```python
from build123d import *

# Parameters (mm, degrees)
SKETCH2_W           = 150
SKETCH2_H           = 260
BOSS_EXTRUDE1_DEPTH = 10
SKETCH3_R           = 3.125
CUT_EXTRUDE1_DEPTH  = 151.416089565
SKETCH4_R           = 5.5
CUT_EXTRUDE2_DEPTH  = 5
SKETCH5_R           = 3.5
CUT_EXTRUDE3_DEPTH  = 151.416089565


with BuildPart() as part:
    # Sketch2 → Boss-Extrude1 (new body)
    with BuildSketch(Plane(origin=(0, 0, 0), x_dir=(1, 0, 0), z_dir=(0, 1, 0))):
        Rectangle(SKETCH2_W, SKETCH2_H)
    extrude(amount=BOSS_EXTRUDE1_DEPTH)

    # Sketch3 → Cut-Extrude1 (cut, through all)
    with BuildSketch(Plane(origin=(0, 10, 0), x_dir=(1, 0, 0), z_dir=(0, 1, 0))):
        with Locations(Location((-54.447222151, -54.447222151, 0), (0, 0, 270))):
            Circle(SKETCH3_R)
        with Locations(Location((-43.840620434, -43.840620434, 0), (0, 0, 270))):
            Circle(SKETCH3_R)
        with Locations(Location((54.447222151, 54.447222151, 0), (0, 0, 270))):
            Circle(SKETCH3_R)
        with Locations(Location((43.840620434, 43.840620434, 0), (0, 0, 270))):
            Circle(SKETCH3_R)
        with Locations(Location((-54.447222151, 54.447222151, 0), (0, 0, 270))):
            Circle(SKETCH3_R)
        with Locations(Location((-43.840620434, 43.840620434, 0), (0, 0, 270))):
            Circle(SKETCH3_R)
        with Locations(Location((54.447222151, -54.447222151, 0), (0, 0, 270))):
            Circle(SKETCH3_R)
        with Locations(Location((43.840620434, -43.840620434, 0), (0, 0, 270))):
            Circle(SKETCH3_R)
    extrude(amount=-CUT_EXTRUDE1_DEPTH, mode=Mode.SUBTRACT)

    # Sketch4 → Cut-Extrude2 (cut, symmetric)
    with BuildSketch(Plane(origin=(0, 10, 0), x_dir=(1, 0, 0), z_dir=(0, 1, 0))):
        with Locations(Location((-43.840620434, -43.840620434, 0), (0, 0, 270))):
            Circle(SKETCH4_R)
        with Locations(Location((-54.447222151, -54.447222151, 0), (0, 0, 270))):
            Circle(SKETCH4_R)
        with Locations(Location((43.840620434, -43.840620434, 0), (0, 0, 270))):
            Circle(SKETCH4_R)
        with Locations(Location((54.447222151, -54.447222151, 0), (0, 0, 270))):
            Circle(SKETCH4_R)
        with Locations(Location((43.840620434, 43.840620434, 0), (0, 0, 270))):
            Circle(SKETCH4_R)
        with Locations(Location((54.447222151, 54.447222151, 0), (0, 0, 270))):
            Circle(SKETCH4_R)
        with Locations(Location((-43.840620434, 43.840620434, 0), (0, 0, 270))):
            Circle(SKETCH4_R)
        with Locations(Location((-54.447222151, 54.447222151, 0), (0, 0, 270))):
            Circle(SKETCH4_R)
    extrude(amount=CUT_EXTRUDE2_DEPTH, both=True, mode=Mode.SUBTRACT)

    # Sketch5 → Cut-Extrude3 (cut, through all)
    with BuildSketch(Plane(origin=(0, 10, 0), x_dir=(1, 0, 0), z_dir=(0, 1, 0))):
        with Locations(Location((-65, 115, 0), (0, 0, 270))):
            Circle(SKETCH5_R)
        with Locations(Location((-39.6, 115, 0), (0, 0, 270))):
            Circle(SKETCH5_R)
        with Locations(Location((-14.2, 115, 0), (0, 0, 270))):
            Circle(SKETCH5_R)
        with Locations(Location((11.2, 115, 0), (0, 0, 270))):
            Circle(SKETCH5_R)
        with Locations(Location((36.6, 115, 0), (0, 0, 270))):
            Circle(SKETCH5_R)
        with Locations(Location((62, 115, 0), (0, 0, 270))):
            Circle(SKETCH5_R)
        with Locations(Location((-65, -113.6, 0), (0, 0, 270))):
            Circle(SKETCH5_R)
        with Locations(Location((-39.6, -113.6, 0), (0, 0, 270))):
            Circle(SKETCH5_R)
        with Locations(Location((-14.2, -113.6, 0), (0, 0, 270))):
            Circle(SKETCH5_R)
        with Locations(Location((11.2, -113.6, 0), (0, 0, 270))):
            Circle(SKETCH5_R)
        with Locations(Location((36.6, -113.6, 0), (0, 0, 270))):
            Circle(SKETCH5_R)
        with Locations(Location((62, -113.6, 0), (0, 0, 270))):
            Circle(SKETCH5_R)
    extrude(amount=-CUT_EXTRUDE3_DEPTH, mode=Mode.SUBTRACT)


solid = part.part
```
Input: part model. Units: mm. Frame: model coordinates. A direction names the side the tool comes from. Coordinates: 2 decimals unless noted, no trailing zeros. Write each loop counter-clockwise with the first axis right and the second up, starting at its lowest first coordinate (ties: lowest second). Pieces come first, ordered by that corner, then holes. Notation, with made-up numbers: (-8, 11) -> (2, 11) arc R26 cw to (2, 33) -> close; hole circle Ø6 at (31.5, 53.25). An arc over 180 degrees is marked (long way). Answer as a JSON object with one key per item and string values.
1. Mould query, pull axis X, two halves, no side actions, for faces 1 (the face through (-1, 10, -2)), 2 (the face through (62.154, 5.07, 110.103)), 3 (the face through (75, 5, 2)), 4 (the face through (-75, 5, 2)). Classes: released by +X, released by -X, zero draft, split by the parting line, or undercut.
Result set:
{"face 1": "zero draft", "face 2": "undercut", "face 3": "released by +X", "face 4": "released by -X"}
2. Section B-B on z = -115. Return the cut outline in (x, y), then the cut area to 3 significant figures.
Result set:
{"outline": "(-75, 0) -> (-68.5, 0) -> (-68.5, 10) -> (-75, 10) -> close; (-61.5, 0) -> (-43.1, 0) -> (-43.1, 10) -> (-61.5, 10) -> close; (-36.1, 0) -> (-17.7, 0) -> (-17.7, 10) -> (-36.1, 10) -> close; (-10.7, 0) -> (7.7, 0) -> (7.7, 10) -> (-10.7, 10) -> close; (14.7, 0) -> (33.1, 0) -> (33.1, 10) -> (14.7, 10) -> close; (40.1, 0) -> (58.5, 0) -> (58.5, 10) -> (40.1, 10) -> close; (65.5, 0) -> (75, 0) -> (75, 10) -> (65.5, 10) -> close", "area": "1,080 mm2"}
3. Section C-C on y = 2.25. Count the separate pieces of the cut face and the enclosed holes in it, then the cut area to 3 significant figures.
Result set:
{"separate pieces": "1", "enclosed holes": "20", "area": "38,300 mm2"}
4. Section A-A on x = 11.2. Return the cut outline in (y, z), then the cut area to 3 significant figures.
Result set:
{"outline": "(0, -130) -> (10, -130) -> (10, -118.5) -> (0, -118.5) -> close; (0, -111.5) -> (10, -111.5) -> (10, 110.1) -> (0, 110.1) -> close; (0, 117.1) -> (10, 117.1) -> (10, 130) -> (0, 130) -> close", "area": "2,460 mm2"}
5. Material intervals for line 1 (X direction, y = 6.5, z = 43.5); line 2 (Z direction, x = -62.5, y = 7); line 3 (Z direction, x = 42, y = 3.5), sorted ascending. Write a range as from..to.
Result set:
{"line 1": "x = -75..-49.33, -38.35..38.35, 49.33..75", "line 2": "z = -130..-117.45, -112.55..111.15, 116.05..130", "line 3": "z = -130..-46.37, -41.32..41.32, 46.37..130"}
6. First-contact query: P1, Ø9, axis at x = 44.5, z = -43.5, coming from the +Y side. Flat tip, straight axial feed; report the tip coordinate or a pass-through.
Result set:
{"P1": "stops at y = 5"}
7. Access query for faces 5 (the face through (-64.846, 5.07, 110.103)), 6 (the face through (51.1, 7.54, -58.81)). Directions: +Z, -Z, +X, -X, +Y, -Y. A direction counts if a zero-diameter tool reaches every point of the face in a straight line with its end or side. Return the directions, or none.
Result set:
{"face 5": "+Y, -Y", "face 6": "+Y"}
